```python
from build123d import *

# Parameters (mm, degrees)
SKETCH1_R           = 0.75
BOSS_EXTRUDE1_DEPTH = 12
SKETCH1_3_R         = 1.5
SKETCH1_3_R_2       = 0.75
BOSS_EXTRUDE2_DEPTH = 5
BOSS_EXTRUDE3_START = -2
SKETCH1_4_R         = 2.5
SKETCH1_4_R_2       = 1.5
SKETCH1_4_R_3       = 0.75
BOSS_EXTRUDE3_DEPTH = 2


with BuildPart() as part:
    # Sketch1 → Boss-Extrude1 (new body)
    with BuildSketch(Plane.XY):
        Circle(SKETCH1_R)
    extrude(amount=BOSS_EXTRUDE1_DEPTH)

    # Sketch1_3 → Boss-Extrude2 (add)
    with BuildSketch(Plane.XY):
        Circle(SKETCH1_3_R)
        Circle(SKETCH1_3_R_2, mode=Mode.SUBTRACT)
    extrude(amount=BOSS_EXTRUDE2_DEPTH)

    # Sketch1_4 → Boss-Extrude3 (add)
    # profile 1 of 3: a face of its own
    with BuildSketch(Plane.XY.offset(BOSS_EXTRUDE3_START)):
        Circle(SKETCH1_4_R)
        Circle(SKETCH1_4_R_2, mode=Mode.SUBTRACT)
    # profile 2 of 3: a face of its own
    with BuildSketch(Plane.XY.offset(BOSS_EXTRUDE3_START)):
        Circle(SKETCH1_4_R_2)
        Circle(SKETCH1_4_R_3, mode=Mode.SUBTRACT)
    # profile 3 of 3: a face of its own
    with BuildSketch(Plane.XY.offset(BOSS_EXTRUDE3_START)):
        Circle(SKETCH1_4_R_3)
    extrude(amount=BOSS_EXTRUDE3_DEPTH)


solid = part.part
```
Part model, mm, in its own coordinate system. A direction names the side the tool comes from. Coordinates: 2 decimals unless noted, no trailing zeros. Write each loop counter-clockwise with the first axis right and the second up, starting at its lowest first coordinate (ties: lowest second). Pieces come first, ordered by that corner, then holes.
Item 1: Mould opens along Z. For faces 1 (the face through (0, -2, 0)), 2 (the face through (0, 0, -2)), 3 (the face through (-1.5, 0.07, 2.46)) say: released by +Z, released by -Z, zero draft, split by the parting line, or undercut.
Item 2: Slice it at C-C (z = 10.5). Write the cut outline in (x, y).
Item 3: Probe line 1 (Z direction, x = -0.7, y = -2); line 2 (X direction, y = -0.1, z = 3.25). List the from-to ranges inside material, lowest first.
Item 4: Slice it at D-D (y = -1.35). Write the cut outline in (x, z), and give its area (3 significant figures).
Item 5: Slice it at A-A (x = 0). Write the cut outline in (y, z).
Item 6: Which spindle directions (+Z, -Z, +X, -X, +Y, -Y) get a long thin tool onto all of the face, cutting with end or side? Do faces 4 (the face through (-0.75, 0.03, 8.45)), 5 (the face through (-0.54, -2.44, -1.01)). Say none if no direction does.
Results found:
1. face 1: released by +Z
1. face 2: released by -Z
1. face 3: zero draft
2. outline: circle Ø1.5 at (0, 0)
3. line 1: z = -2 to 0
3. line 2: x = -1.5 to 1.5
4. outline: (-2.1, -2) - (2.1, -2) - (2.1, 0) - (0.65, 0) - (0.65, 5) - (-0.65, 5) - (-0.65, 0) - (-2.1, 0) - close
4. area: 15.0 mm2
5. outline: (-2.5, -2) - (2.5, -2) - (2.5, 0) - (1.5, 0) - (1.5, 5) - (0.75, 5) - (0.75, 12) - (-0.75, 12) - (-0.75, 5) - (-1.5, 5) - (-1.5, 0) - (-2.5, 0) - close
6. face 4: +Z
6. face 5: +Z, -Z
